The model under review builds one solid part; all positions refer to its coordinate system, in mm. Round coordinates to 2 decimals unless told otherwise and drop trailing zeros. Write each question's results on one line, items separated by ' | '.
```python
from build123d import *

# Parameters (mm, degrees)
SKETCH1_R                             = 79.375
BOSS_EXTRUDE1_DEPTH                   = 3.175
TAP_DRILL_FOR_M5X0_8_TAP1_D           = 4.2
TAP_DRILL_FOR_M7X1_0_TAP1_D           = 6
SKETCH32_R                            = 4.127000001
CUT_EXTRUDE1_DEPTH                    = 113.432663181
SKETCH32_4_R                          = 11.126999971
SKETCH32_4_R_2                        = 4.127000001
CUT_EXTRUDE2_DEPTH                    = 4.35
CHAMFER1_SIZE                         = 4.35
TAP_DRILL_FOR_M2X0_4_TAP1_D           = 1.6
TAP_DRILL_FOR_M2X0_4_TAP1_CSINK_D     = 1.65
TAP_DRILL_FOR_M2X0_4_TAP1_CSINK_ANGLE = 90
CHAMFER2_SIZE                         = 2.5
TAP_DRILL_FOR_M5X0_8_TAP2_D           = 4.2


with BuildPart() as part:
    # Sketch1 → Boss-Extrude1 (new, symmetric)
    with BuildSketch(Plane(origin=(0, 0, 0), x_dir=(1, 0, 0), z_dir=(0, 1, 0))):
        with Locations(Location((0, 0, 0), (0, 0, 270))):
            Circle(SKETCH1_R)
    extrude(amount=BOSS_EXTRUDE1_DEPTH, both=True)

    # Tap Drill for M5x0.8 Tap1 (through all)
    with Locations(Plane(origin=(0, 3.175, 0), x_dir=(1, 0, 0), z_dir=(0, 1, 0))):
        with Locations((-27.3188086, 41.38978387), (4.4311914, 41.38978387), (-15.875, -12.895910708), (15.875, -12.895910708)):
            Hole(TAP_DRILL_FOR_M5X0_8_TAP1_D / 2)

    # Tap Drill for M7x1.0 Tap1 (through all)
    with Locations(Plane(origin=(0, 3.175, 0), x_dir=(1, 0, 0), z_dir=(0, 1, 0))):
        with Locations((-44.245, 9.941583672), (-44.245, -15.058416328), (44.245, 9.941583672), (44.245, -15.058416328)):
            Hole(TAP_DRILL_FOR_M7X1_0_TAP1_D / 2)

    # Sketch32 → Cut-Extrude1 (cut, through all)
    with BuildSketch(Plane(origin=(0, 3.175, 0), x_dir=(1, 0, 0), z_dir=(0, 1, 0))):
        with Locations(Location((0, 0, 0), (0, 0, 270))):
            Circle(SKETCH32_R)
    extrude(amount=-CUT_EXTRUDE1_DEPTH, mode=Mode.SUBTRACT)

    # Sketch32<4> → Cut-Extrude2 (cut)
    with BuildSketch(Plane(origin=(0, 3.175, 0), x_dir=(1, 0, 0), z_dir=(0, 1, 0))):
        with Locations(Location((0, 0, 0), (0, 0, 270))):
            Circle(SKETCH32_4_R)
        with Locations(Location((0, 0, 0), (0, 0, 270))):
            Circle(SKETCH32_4_R_2, mode=Mode.SUBTRACT)
    extrude(amount=-CUT_EXTRUDE2_DEPTH, mode=Mode.SUBTRACT)

    # Chamfer1
    chamfer1_edges = [part.edges().sort_by_distance(p)[0] for p in [
        (0, 3.175, -11.126999971),
    ]]
    chamfer(chamfer1_edges, length=CHAMFER1_SIZE - 0.0001)  # a hair under: the kernel refuses the full size

    # Tap Drill for M2x0.4 Tap1 (through all)
    with Locations(Plane(origin=(0, -1.175, 0), x_dir=(1, 0, 0), z_dir=(0, 1, 0))):
        with Locations((-8, 0), (-5.656854249, 5.656854249), (0, 8), (5.656854249, 5.656854249), (8, 0), (5.656854249, -5.656854249), (0, -8), (-5.656854249, -5.656854249)):
            CounterSinkHole(TAP_DRILL_FOR_M2X0_4_TAP1_D / 2, TAP_DRILL_FOR_M2X0_4_TAP1_CSINK_D / 2, counter_sink_angle=TAP_DRILL_FOR_M2X0_4_TAP1_CSINK_ANGLE)

    # Chamfer2
    chamfer2_edges = [part.edges().sort_by_distance(p)[0] for p in [
        (0, 3.175, -79.375),
    ]]
    chamfer(chamfer2_edges, length=CHAMFER2_SIZE)

    # Tap Drill for M5x0.8 Tap2 (through all)
    with Locations(Plane(origin=(0, 3.175, 0), x_dir=(1, 0, 0), z_dir=(0, 1, 0))):
        with Locations((-57.723385101, 0), (0, 57.723385101), (57.723385101, 0), (0, -57.723385101)):
            Hole(TAP_DRILL_FOR_M5X0_8_TAP2_D / 2)


solid = part.part
```
Q1. Insertion check: P1, Ø1, axis at y = -1.5, z = 58, coming from the +X side; P2, Ø2.5, axis at x = 8, z = 0, coming from the -Y side (3 decimals); P3, Ø18, axis at x = 0, z = 0, coming from the +Y side (3 decimals); P4, Ø1.5, axis at y = 0.5, z = -23.5, coming from the -X side. Each pin has a flat end and moves straight along its axis. Give the tip position at first contact, or say it passes through.
Evaluation:
P1: stops at x = 54.72 | P2: stops at y = -3.175 | P3: stops at y = -1.175 | P4: stops at x = -76.04
Q2. For probe 1 along Z at (x, y) = (44.5, -2.25); probe 2 along Z at (x, y) = (-8, -2.25); probe 3 along Z at (x, y) = (-9.5, -0.75), list the stretches that pass through material, from the lowest coordinate up.
Evaluation:
probe 1: z = -65.73 to -12.93, -6.95 to 12.07, 18.05 to 65.73 | probe 2: z = -78.97 to -0.8, 0.8 to 78.97 | probe 3: z = -78.8 to -6.57, 6.57 to 78.8
Q3. We need section A-A (x = 44). State how many separate pieces and enclosed holes the cut face has, plus the area to 3 significant figures.
Evaluation:
separate pieces: 3 | enclosed holes: 0 | area: 756 mm^2
Q4. The part is to be moulded in two halves that separate along X. For faces 1 (the cylindrical face through (44.895, -0.044, 17.987)), 2 (the cylindrical face through (23.84, -1.22, 75.71)), 3 (the flat face through (-16, 3.175, -1)), 4 (the cylindrical face through (-25.652, -0.044, -40.112)), say which applies: released by +X, released by -X, zero draft, split by the parting line, or undercut.
Evaluation:
face 1: undercut | face 2: split by the parting line | face 3: zero draft | face 4: undercut
